from build123d import *

# Parameters (mm, degrees)
SKETCH1_R           = 0.775
BOSS_EXTRUDE1_DEPTH = 2
SKETCH2_R           = 0.95
SKETCH2_W           = 8
SKETCH2_H           = 11
SKETCH2_W_2         = 8.8
SKETCH2_H_2         = 11.4
SKETCH2_W_3         = 2
SKETCH2_H_3         = 3.5
SKETCH2_W_4         = 2.5
SKETCH2_H_4         = 6.5
CUT_EXTRUDE1_DEPTH  = 3
FILLET1_R           = 2
SKETCH3_R           = 1.275
CUT_EXTRUDE2_DEPTH  = 0.5


with BuildPart() as part:
    # Sketch1 → Boss-Extrude1 (new body)
    with BuildSketch(Plane(origin=(0, 0, 0), x_dir=(1, 0, 0), z_dir=(0, 1, 0))):
        Polygon((18.486983138, -44.730983302), (23.486983138, -44.730983302), (23.486983138, 1.269016698), (18.486983138, 1.269016698), (18.486983138, -3.730983302), (-0.513016862, -3.730983302), (-0.513016862, 1.269016698), (-5.513016862, 1.269016698), (-5.513016862, -39.730983302), (-0.513016862, -39.730983302), (18.486983138, -39.730983302), align=None)
        with Locations((-3.013016862, -1.230983302)):
            Circle(SKETCH1_R, mode=Mode.SUBTRACT)
        with Locations((20.986983138, -1.230983302)):
            Circle(SKETCH1_R, mode=Mode.SUBTRACT)
        with Locations((20.986983138, -42.230983302)):
            Circle(SKETCH1_R, mode=Mode.SUBTRACT)
    extrude(amount=BOSS_EXTRUDE1_DEPTH)

    # Sketch2 → Cut-Extrude1 (cut, through all)
    with BuildSketch(Plane(origin=(0, 2, 0), x_dir=(1, 0, 0), z_dir=(0, 1, 0))):
        with Locations((17.586983138, -14.730983302)):
            Circle(SKETCH2_R)
        with Locations((17.586983138, -30.130983302)):
            Circle(SKETCH2_R)
        with Locations((5.486983138, -9.230983302)):
            Rectangle(SKETCH2_W, SKETCH2_H)
        with Locations((19.086983138, -22.430983302)):
            Rectangle(SKETCH2_W_2, SKETCH2_H_2)
        with Locations((4.836983138, -17.280983302)):
            Rectangle(SKETCH2_W_3, SKETCH2_H_3)
        with Locations((0.286983138, -31.380983302)):
            Rectangle(SKETCH2_W_4, SKETCH2_H_4)
    extrude(amount=-CUT_EXTRUDE1_DEPTH, mode=Mode.SUBTRACT)

    # Fillet1
    fillet1_edges = [part.edges().sort_by_distance(p)[0] for p in [
        (-5.513016862, 1, -1.269016698),
        (-0.513016862, 1, -1.269016698),
        (18.486983138, 1, -1.269016698),
        (23.486983138, 1, -1.269016698),
        (23.486983138, 1, 44.730983302),
        (18.486983138, 1, 44.730983302),
    ]]
    fillet(fillet1_edges, radius=FILLET1_R)

    # Sketch3 → Cut-Extrude2 (cut)
    with BuildSketch(Plane(origin=(0, 2, 0), x_dir=(1, 0, 0), z_dir=(0, 1, 0))):
        with Locations((-3.013016862, -1.230983302)):
            Circle(SKETCH3_R)
        with Locations((20.986983138, -1.230983302)):
            Circle(SKETCH3_R)
        with Locations((20.986983138, -42.230983302)):
            Circle(SKETCH3_R)
    extrude(amount=-CUT_EXTRUDE2_DEPTH, mode=Mode.SUBTRACT)


solid = part.part
Work out the finished part from the listing and answer in its coordinate system (mm). A direction names the side the tool comes from. Give positions to 0.01 mm unless a question says otherwise; leave off trailing zeros. Order: outer loops, then holes, each group sorted by start corner. A loop starts at its lowest first (then second) coordinate and runs counter-clockwise, first axis right, second up. Notation, with made-up numbers: (63, 16.25) -> (116, 16.25) arc R24 cw to (116, 35.25) -> close; hole circle Ø4 at (-10.5, 38.25). An arc over 180 degrees is marked (long way). Answer as a JSON object with one key per item and string values. Group by question number.
1. Section A-A on z = 4.5 is taken. Determine the outline of the cut face in (x, y), plus the area to 3 significant figures.
2. Section C-C on x = 7 is taken. Determine the outline of the cut face in (y, z).
3. Section D-D on y = 1 is taken. Count the separate pieces of the cut face and the enclosed holes in it, plus the area to 3 significant figures.
4. Consider line 1 along X through (y, z) = (0.8, 13); line 2 along Z through (x, y) = (16.5, 1.5); line 3 along X through (y, z) = (0.8, 34). Determine where each line is inside the solid, lowest interval first. Write a range as [from, to].
5. Section B-B on x = 16 is taken. Determine the outline of the cut face in (y, z).
6. Flat-ended cylindrical pins translate along their axes: pin 1 Ø0.6 at (x, y) = (0.5, 1) entering from +Z; pin 2 Ø0.6 at (x, y) = (15.5, 1) entering from -Z; pin 3 Ø3.5 at (x, z) = (20.99, 42.23) entering from -Y; pin 4 Ø1.5 at (x, z) = (17.59, 30.13) entering from +Y. Find the tip coordinate at first contact, or state that the pin passes through.
7. A tool of negligible diameter and unlimited length cuts with its end or side. For faces 4 (the flat face through (18.487, 1, 41)), 5 (the flat face through (5, 1, 19.031)), 6 (the cylindrical face through (19.713, 1.754, 1.175)), from which of +Z, -Z, +X, -X, +Y, -Y can it reach the whole face along a straight path? Write none if from no direction.
8. The mould has two halves that part along Z. Classify faces 1 (the cylindrical face through (18.493, 1.014, 29.846)), 2 (the flat face through (-3, 1, -1.269)), 3 (the flat face through (21, 1, 44.731)): released by +Z, released by -Z, zero draft, split by the parting line, or undercut.
Result sheet:
{
 "1": {"outline": "(-5.51, 0) -> (1.49, 0) -> (1.49, 2) -> (-5.51, 2) -> close; (9.49, 0) -> (23.49, 0) -> (23.49, 2) -> (9.49, 2) -> close", "area": "42.0 mm^2"},
 "2": {"outline": "(0, 14.73) -> (2, 14.73) -> (2, 39.73) -> (0, 39.73) -> close"},
 "3": {"separate pieces": "1", "enclosed holes": "7", "area": "891 mm^2"},
 "4": {"line 1": "x = [-5.51, 1.49], [9.49, 23.49]", "line 2": "z = [3.73, 16.73], [28.13, 39.73]", "line 3": "x = [-5.51, -0.96], [1.54, 23.49]"},
 "5": {"outline": "(0, 3.73) -> (2, 3.73) -> (2, 16.73) -> (0, 16.73) -> close; (0, 28.13) -> (2, 28.13) -> (2, 39.73) -> (0, 39.73) -> close"},
 "6": {"pin 1": "stops at z = 39.73", "pin 2": "stops at z = 3.73", "pin 3": "stops at y = 0", "pin 4": "passes through"},
 "7": {"face 4": "+Z, -X, +Y, -Y", "face 5": "+Y, -Y", "face 6": "+Y"},
 "8": {"face 1": "undercut", "face 2": "released by -Z", "face 3": "released by +Z"}
}
